```python
from build123d import *

# Parameters (mm, degrees)
F1_DEPTH = 6.35


with BuildPart() as f1:
    # F0 (on Top) → F1 (new body)
    with BuildSketch(Plane.XY):
        Polygon((-14.7529365335, 1.3235569542), (-5.8176855718, -13.6218748328), (11.1574091143, -9.7423385914), (12.7133436308, 7.6007784534), (-3.3001306398, 14.4398780166), align=None)
        Polygon((12.7133436308, 7.6007784534), (11.1574091143, -9.7423385914), (38.6236892786, -3.4651170922), align=None)
        Polygon((-5.8176855718, -13.6218748328), (8.6398541823, -37.8040914407), (11.1574091143, -9.7423385914), align=None)
        Polygon((-33.2839657361, -19.899096332), (-5.8176855718, -13.6218748328), (-14.7529365335, 1.3235569542), align=None)
        Polygon((-29.2104762876, 25.5057735621), (-14.7529365335, 1.3235569542), (-3.3001306398, 14.4398780166), align=None)
        Polygon((-3.3001306398, 14.4398780166), (12.7133436308, 7.6007784534), (15.2308985628, 35.6625313028), align=None)
    extrude(amount=F1_DEPTH)


solid = f1.part
```
Geometry: final body of the model. Coordinates: model frame, mm. A direction names the side the tool comes from. Coordinates: 2 decimals unless noted, no trailing zeros. Order: outer loops, then holes, each group sorted by start corner. A loop starts at its lowest first (then second) coordinate and runs counter-clockwise, first axis right, second up. Notation, with made-up numbers: (10.25, 18.25) - (34.25, 18.25) arc R20 cw to (34.25, 47.25) - close; hole circle Ø7 at (60.25, 27.25). An arc over 180 degrees is marked (long way). Write each question's results on one line, items separated by ' | '.
(1) First-contact query: pin 1 Ø1 at (y, z) = (-19, 3.5) entering from +X; pin 2 Ø3 at (y, z) = (4.5, 1) entering from -X; pin 3 Ø1.5 at (x, z) = (-25, 5.5) entering from -Y. Flat tips, straight axial feed; report the tip coordinate or a pass-through.
Values found:
pin 1: stops at x = 10.37 | pin 2: stops at x = -17.55 | pin 3: stops at y = -18.18
(2) Section query B-B, the plane y = -19. Return the cut outline in (x, z).
Values found:
outline: (-32.5, 0) - (-29.35, 0) - (-29.35, 6.35) - (-32.5, 6.35) - close; (-2.6, 0) - (10.33, 0) - (10.33, 6.35) - (-2.6, 6.35) - close
(3) Section query C-C, the plane y = 18. Return the cut outline in (x, z).
Values found:
outline: (-24.72, 0) - (-11.64, 0) - (-11.64, 6.35) - (-24.72, 6.35) - close; (-0.19, 0) - (13.65, 0) - (13.65, 6.35) - (-0.19, 6.35) - close
(4) Set-up query: faces 4 (the face through (-19.743, -16.804, 3.131)), 5 (the face through (-16.074, 19.895, 3.131)), 6 (the face through (3, 2, 6.35)), 7 (the face through (-22.08, 13.58, 3.13)), 8 (the face through (13.954, 21.435, 3.131)). Return all of +Z, -Z, +X, -X, +Y, -Y with unobstructed straight access to the full face (end or side cutting, diameter ignored); none if empty.
Values found:
face 4: +Z, -Z, -Y | face 5: +Z, -Z, +Y | face 6: +Z, +X, -X, +Y, -Y | face 7: +Z, -Z, -X | face 8: +Z, -Z, +X
(5) Line query: line 1 (Y direction, x = -24.5, z = 3.25); line 2 (Y direction, x = 3, z = 3.25); line 3 (Y direction, x = 17, z = 4.25). Output: solid intervals per line, ascending. Write a range as [from, to].
Values found:
line 1: y = [-17.89, -9.84], [17.63, 23.49] | line 2: y = [-28.37, 21.66] | line 3: y = [-8.41, 5.77]
(6) Section query D-D, the plane x = 5. Return the cut outline in (y, z).
Values found:
outline: (-31.72, 0) - (23.95, 0) - (23.95, 6.35) - (-31.72, 6.35) - close
(7) Mould query, pull axis Y, two halves, no side actions, for faces 1 (the face through (1.31, -25.544, 3.131)), 2 (the face through (3, 2, 0)), 3 (the face through (-23.89, -9.14, 3.13)). Classes: +Y half, -Y half, draft (parallel to the pull), parting line (faces both ways), or undercut.
Values found:
face 1: -Y half | face 2: draft | face 3: undercut
(8) Section query A-A, the plane z = 1.25. Return the cut outline in (x, y), plus the area to 3 significant figures.
Values found:
outline: (-33.28, -19.9) - (-5.82, -13.62) - (8.64, -37.8) - (11.16, -9.74) - (38.62, -3.47) - (12.71, 7.6) - (15.23, 35.66) - (-3.3, 14.44) - (-29.21, 25.51) - (-14.75, 1.32) - close | area: 1,690 mm²
